Solid Edge part; units mm, degrees
sketch "Sketch1" plane through (0, 0, 0) normal (0, -1, 0) x (1, 0, 0)
  circle A0 centre (13.8386, 9.2832) radius 8
  circle A1 centre (13.8386, 9.2832) radius 3
extrude "Protrusion1" add sketch "Sketch1" along normal blind 1.1
sketch "Sketch2" plane through (13.8386, -1.1, 9.2832) normal (0, -1, 0) x (1, 0, 0)
  circle A0 centre (0, 0) radius 4.6
  circle A1 centre (0, 0) radius 6.11
extrude "ExtrudedProtrusion_2" add sketch "Sketch2" along normal blind 3.8
sketch "Sketch3" plane through (13.8386, -1.1, 9.2832) normal (0, -1, 0) x (1, 0, 0)
  circle A0 centre (0, 0) radius 3
  circle A1 centre (0, 0) radius 4.6
extrude "ExtrudedProtrusion_3" add sketch "Sketch3" along normal blind 1.4
Could you check a few things on this model? Use its own coordinates, in mm. A direction names the side the tool comes from. Round coordinates to 2 decimals unless told otherwise and drop trailing zeros. Loops run counter-clockwise (first coordinate to the right, second up) from the corner with the lowest first, then second, coordinate; pieces in that order, holes last.
Q1. I want a section at C-C (y = -0.75). Write out the boundary of the cut face in (x, z).
Q2. For P1, Ø1.5, axis at y = -0.5, z = 15, coming from the -X side; P2, Ø1, axis at y = -3, z = 8, coming from the +X side; P3, Ø1.5, axis at x = 10.5, y = -3.5, coming from the +Z side, each with a flat end and sliding along its axis, tell me the tip position at first contact or that it passes through.
Q3. I want a section at B-B (z = 11.25). Write out the boundary of the cut face in (x, y).
Q4. Please list where these lines run through material, in increasing order: L1, parallel to X at y = -1.95, z = 9.25; L2, parallel to Y at x = 11.25, z = 3.5; L3, parallel to Z at x = 16, y = -4.6.
Q5. On a 3-axis mill with a long thin cutter (end or side, diameter ignored), from which of +Z, -Z, +X, -X, +Y, -Y can I reach the whole of each face in a straight line? I mean faces 4 (the flat face through (18, -4.9, 12)), 5 (the cylindrical face through (18.088, -3.683, 11.045)). Say none if no direction works.
Q6. Thinking about a two-plate mould opening in X: for faces 1 (the flat face through (11, -1.1, 15)), 2 (the cylindrical face through (19.666, -2.973, 7.448)), 3 (the flat face through (14, -2.5, 6)), which applies, pulls with the +X half, pulls with the -X half, needs draft (parallel to the pull), parting line crosses it, or undercut?
Q7. I want a section at A-A (x = 12). Write out the boundary of the cut face in (y, z), and give its area (3 significant figures).
Q8. I want a section at D-D (z = 13). Write out the boundary of the cut face in (x, y).
Answer below:
1. outline: circle Ø16 at (13.84, 9.28); hole circle Ø6 at (13.84, 9.28)
2. P1: stops at x = 7.57
2. P2: stops at x = 19.9
2. P3: stops at z = 14.82
3. outline: (6.08, -1.1) - (8.05, -1.1) - (8.05, -4.9) - (9.68, -4.9) - (9.68, -2.5) - (11.57, -2.5) - (11.57, 0) - (6.08, 0) - close; (16.1, -2.5) - (18, -2.5) - (18, -4.9) - (19.62, -4.9) - (19.62, -1.1) - (21.59, -1.1) - (21.59, 0) - (16.1, 0) - close
4. L1: x = 7.73 to 10.84, 16.84 to 19.95
4. L2: y = -1.1 to 0
4. L3: z = 3.57 to 5.22, 13.34 to 15
5. face 4: +Z, -Z, +X, -X, -Y
5. face 5: -Y
6. face 1: needs draft
6. face 2: parting line crosses it
6. face 3: undercut
7. outline: (-4.9, 3.46) - (-1.1, 3.46) - (-1.1, 1.5) - (0, 1.5) - (0, 6.91) - (-2.5, 6.91) - (-2.5, 5.07) - (-4.9, 5.07) - close; (-4.9, 13.5) - (-2.5, 13.5) - (-2.5, 11.65) - (0, 11.65) - (0, 17.07) - (-1.1, 17.07) - (-1.1, 15.11) - (-4.9, 15.11) - close
7. area: 29.3 mm2
8. outline: (6.75, -1.1) - (8.99, -1.1) - (8.99, -4.9) - (11.13, -4.9) - (11.13, -2.5) - (16.55, -2.5) - (16.55, -4.9) - (18.69, -4.9) - (18.69, -1.1) - (20.92, -1.1) - (20.92, 0) - (6.75, 0) - close
